```python
from build123d import *

# Parameters (mm, degrees)
BOSS_EXTRUDE1_DEPTH = 4.826
FILLET1_R           = 1.27
FILLET2_R           = 2.54


with BuildPart() as part:
    # Sketch1 → Boss-Extrude1 (new body)
    with BuildSketch(Plane(origin=(0, 0, 0), x_dir=(1, 0, 0), z_dir=(0, 1, 0))):
        Polygon((-56.134, 29.083), (-40.894, 29.083), (-47.241885042, 18.083256572), (-43.685885042, 16.624574128), (-37.338, 29.083), (-12.7, 29.083), (-12.7, 37.719), (12.7, 37.719), (12.7, 29.083), (37.338, 29.083), (43.685885042, 16.624574128), (47.241885042, 18.083256572), (40.894, 29.083), (56.134, 29.083), (56.134, 16.383), (63.5, 16.383), (63.5, -9.230617291), (56.134, -9.230617291), (56.134, -29.083), (56.134, -30.353), (40.894, -30.353), (40.894, -21.717), (-40.894, -21.717), (-40.894, -30.353), (-56.134, -30.353), (-56.134, -29.083), (-56.134, -9.230617291), (-63.5, -9.230617291), (-63.5, 16.383), (-56.134, 16.383), align=None)
    extrude(amount=BOSS_EXTRUDE1_DEPTH)

    # Fillet1
    fillet1_edges = [part.edges().sort_by_distance(p)[0] for p in [
        (-47.241885042, 2.413, -18.083256572),
        (-43.685885042, 2.413, -16.624574128),
        (43.685885042, 2.413, -16.624574128),
        (47.241885042, 2.413, -18.083256572),
    ]]
    fillet(fillet1_edges, radius=FILLET1_R)

    # Fillet2
    fillet2_edges = [part.edges().sort_by_distance(p)[0] for p in [
        (-40.894, 2.413, -29.083),
        (-37.338, 2.413, -29.083),
        (37.338, 2.413, -29.083),
        (40.894, 2.413, -29.083),
    ]]
    fillet(fillet2_edges, radius=FILLET2_R)


solid = part.part
```
Geometry check sheet. Reference: the model listing, model coordinates, mm. A direction names the side the tool comes from. Coordinates: 2 decimals unless noted, no trailing zeros. Loops run counter-clockwise (first coordinate to the right, second up) from the corner with the lowest first, then second, coordinate; pieces in that order, holes last. Notation, with made-up numbers: (86.5, 29) - (90.5, 29) arc R12 ccw to (90.5, 44) - close; hole circle Ø11 at (-21, 81.5). An arc over 180 degrees is marked (long way). One line per item, written item: value. Start each with the question number.
(1) Tool access check on faces 1 (the flat face through (44.828, 2.379, -22.266)), 2 (the flat face through (60, 2, 9.231)), 3 (the flat face through (56.134, 2, -23)), 4 (the flat face through (-56.134, 2, -23)), 5 (the flat face through (-40.894, 2, 26)). Record the directions out of +Z, -Z, +X, -X, +Y, -Y that give a thin tool (end or side, any length) a straight path to the whole face; none if there is none.
(2) Material ranges on line 1 (X direction, y = 1.1, z = 22); line 2 (X direction, y = 3.15, z = 9.5); line 3 (Z direction, x = -16, y = 3.4), recorded low to high. Write a range as [from, to].
(3) Mould release check, pull along Z, two halves, no side actions. Record for faces 6 (the cylindrical face through (43.074, 2.447, -27.781)), 7 (the flat face through (-24, 2, -29.083)), 8 (the flat face through (12.7, 2, -33)): released by +Z, released by -Z, zero draft, split by the parting line, or undercut.
(4) Cross-section at C-C on z = 12. Enter the section's corners in (x, y), plus the area to 3 significant figures.
(5) Cross-section at A-A on z = -23. Enter the section's corners in (x, y).
(6) Cross-section at B-B on x = -50.5. Enter the section's corners in (y, z).
(7) Depth check by flat-ended pin: P1, Ø1.4, axis at x = 53, y = 3, coming from the -Z side; P2, Ø2.5, axis at y = 3, z = 25, coming from the -X side; P3, Ø3, axis at x = 2.5, z = 20, coming from the -Y side; P4, Ø1.4, axis at y = 1.5, z = -32, coming from the -X side. Enter the tip coordinate at first touch or a pass-through.
Results below:
1. face 1: +Y, -Y
1. face 2: +Z, +X, +Y, -Y
1. face 3: -Z, +X, +Y, -Y
1. face 4: -Z, -X, +Y, -Y
1. face 5: +Z, +Y, -Y
2. line 1: x = [-56.13, -40.89], [40.89, 56.13]
2. line 2: x = [-56.13, 56.13]
2. line 3: z = [-29.08, 21.72]
3. face 6: undercut
3. face 7: released by -Z
3. face 8: zero draft
4. outline: (-56.13, 0) - (56.13, 0) - (56.13, 4.83) - (-56.13, 4.83) - close
4. area: 542 mm2
5. outline: (-56.13, 0) - (-44.4, 0) - (-44.4, 4.83) - (-56.13, 4.83) - close; (-40.44, 0) - (40.44, 0) - (40.44, 4.83) - (-40.44, 4.83) - close; (44.4, 0) - (56.13, 0) - (56.13, 4.83) - (44.4, 4.83) - close
6. outline: (0, -29.08) - (4.83, -29.08) - (4.83, 30.35) - (0, 30.35) - close
7. P1: stops at z = -29.08
7. P2: stops at x = -56.13
7. P3: stops at y = 0
7. P4: stops at x = -12.7
